Here's the drawing with two shaded views (mm, measured from the low corner). I have some questions. A direction names the side the tool comes from. Give positions to 0.01 mm unless a question says otherwise; leave off trailing zeros. Loops run counter-clockwise (first coordinate to the right, second up) from the corner with the lowest first, then second, coordinate; pieces in that order, holes last. Notation, with made-up numbers: (16, 54) - (42, 54) arc R29 ccw to (42, 74) - close; hole circle Ø10 at (-33, 48.5). An arc over 180 degrees is marked (long way). Answer as a JSON object with one key per item and string values. Group by question number.
Item 1: Please list where these lines run through material, in increasing order: L1, parallel to Y at x = 8, z = 17.5; L2, parallel to X at y = 31, z = 9.75; L3, parallel to X at y = 27, z = 7.25.
Item 2: Which directions (+Z, -Z, +X, -X, +Y, -Y) give clear straight access to the entire face, cutting with the end or side of a thin tool? Please do the marked faces 1 and 2.
Item 3: Suppose I cut it at C-C on y = 26. Write out the boundary of the cut face in (x, z).
Item 4: Suppose I cut it at B-B on x = 10. Write out the boundary of the cut face in (y, z).
Item 5: Will these pins go through, and if not, where does the flat tip stop? pin 1 (8 mm diameter, centred on y = 13.5, z = 11, fed in from +X); pin 2 (12 mm diameter, centred on x = 6, z = 8, fed in from -Y); pin 3 (8 mm diameter, centred on x = 5, y = 22, fed in from -Z); pin 4 (3 mm diameter, centred on y = 28, z = 17.5, fed in from -X).
Item 6: Suppose I cut it at A-A on z = 10. Write out the boundary of the cut face in (x, y), and give its area (3 significant figures).
Item 7: Suppose I cut it at D-D on y = 9. Write out the boundary of the cut face in (x, z), and give its area (3 significant figures).
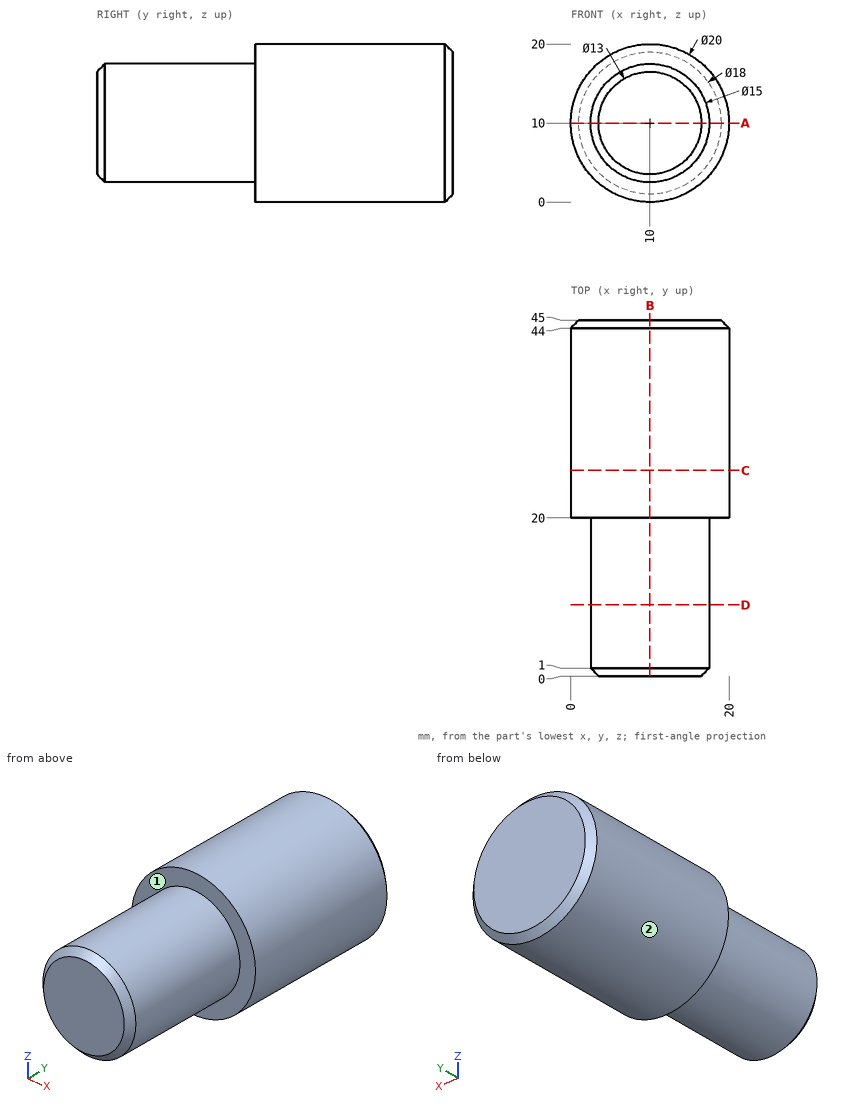
Worked out:
{
 "1": {"L1": "y = 20 to 45", "L2": "x = 0 to 20", "L3": "x = 0.39 to 19.61"},
 "2": {"face 1": "-Y", "face 2": "+Y, -Y"},
 "3": {"outline": "circle Ø20 at (10, 10)"},
 "4": {"outline": "(0, 3.5) - (1, 2.5) - (20, 2.5) - (20, 0) - (44, 0) - (45, 1) - (45, 19) - (44, 20) - (20, 20) - (20, 17.5) - (1, 17.5) - (0, 16.5) - close"},
 "5": {"pin 1": "stops at x = 17.5", "pin 2": "stops at y = 0", "pin 3": "stops at z = 0.05", "pin 4": "stops at x = 2"},
 "6": {"outline": "(0, 20) - (2.5, 20) - (2.5, 1) - (3.5, 0) - (16.5, 0) - (17.5, 1) - (17.5, 20) - (20, 20) - (20, 44) - (19, 45) - (1, 45) - (0, 44) - close", "area": "798 mm2"},
 "7": {"outline": "circle Ø15 at (10, 10)", "area": "177 mm2"}
}
